Check sheet for the drawn part. Datum: minimum x, y, z corner. Units: mm. A direction names the side the tool comes from. Round coordinates to 2 decimals unless told otherwise and drop trailing zeros. Write each loop counter-clockwise with the first axis right and the second up, starting at its lowest first coordinate (ties: lowest second). Pieces come first, ordered by that corner, then holes.
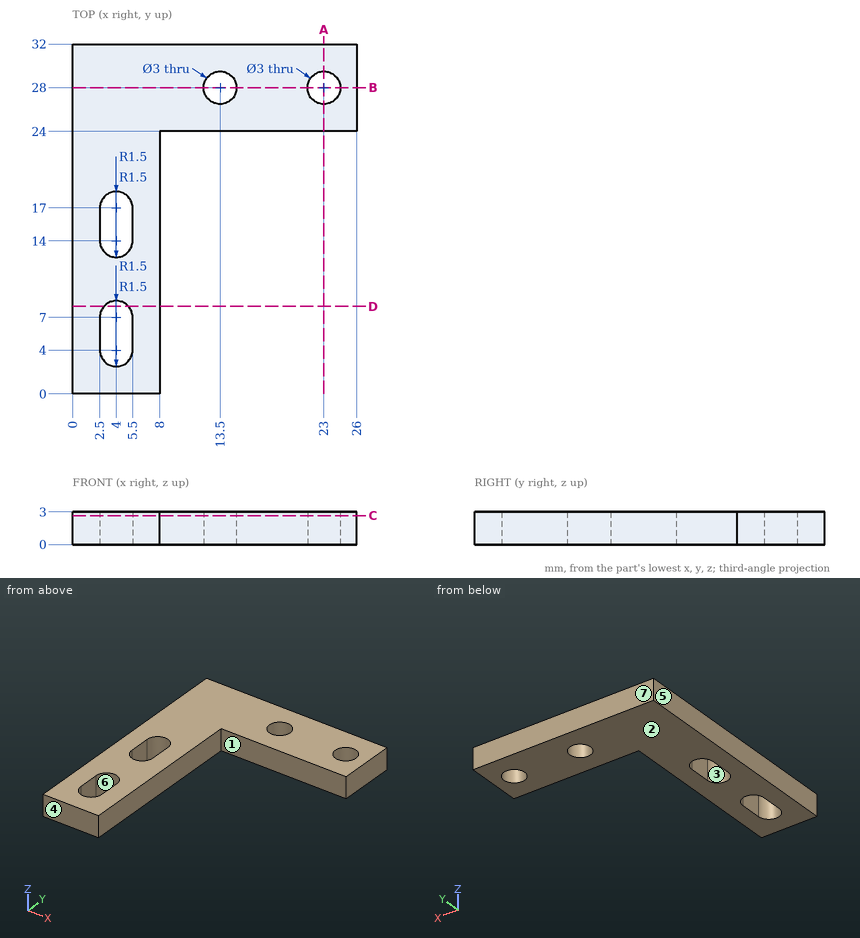
1. Release check for a two-part mould opening along Y. For the marked faces 4, 5, 6 and 7 record: released by +Y, released by -Y, zero draft, split by the parting line, or undercut.
2. Sectioned sample at A-A, the plane x = 23. Enter the section's corners in (y, z), plus the area to 3 significant figures.
3. Scan lines: line 1 along X through (y, z) = (28, 2.2); line 2 along Y through (x, z) = (13.5, 2.1); line 3 along X through (y, z) = (10, 2.25). Record each from-to range of solid material in increasing order.
4. Go/stop test with flat-tipped pins: pin 1 (3.5 mm diameter, centred on x = 13.5, y = 28, fed in from +Z); pin 2 (1.5 mm diameter, centred on y = 5.5, z = 1.5, fed in from +X). Record where each tip stops, or that it passes through.
5. Sectioned sample at B-B, the plane y = 28. Enter the section's corners in (x, z), plus the area to 3 significant figures.
6. Sectioned sample at C-C, the plane z = 2.65. Enter the section's corners in (x, y), plus the area to 3 significant figures.
7. Sectioned sample at D-D, the plane y = 8. Enter the section's corners in (x, z), plus the area to 3 significant figures.
8. Set-up check for the marked faces 1, 2 and 3: record each of +Z, -Z, +X, -X, +Y, -Y from which the full face is reachable in a straight line by a thin tool's end or side.
Computed values:
1. face 4: released by -Y
1. face 5: zero draft
1. face 6: undercut
1. face 7: released by +Y
2. outline: (24, 0) - (26.5, 0) - (26.5, 3) - (24, 3) - close; (29.5, 0) - (32, 0) - (32, 3) - (29.5, 3) - close
2. area: 15.0 mm2
3. line 1: x = 0 to 12, 15 to 21.5, 24.5 to 26
3. line 2: y = 24 to 26.5, 29.5 to 32
3. line 3: x = 0 to 8
4. pin 1: stops at z = 3
4. pin 2: stops at x = 8
5. outline: (0, 0) - (12, 0) - (12, 3) - (0, 3) - close; (15, 0) - (21.5, 0) - (21.5, 3) - (15, 3) - close; (24.5, 0) - (26, 0) - (26, 3) - (24.5, 3) - close
5. area: 60.0 mm2
6. outline: (0, 0) - (8, 0) - (8, 24) - (26, 24) - (26, 32) - (0, 32) - close; hole (2.5, 4) arc R1.5 ccw to (5.5, 4) - (5.5, 7) arc R1.5 ccw to (2.5, 7) - close; hole (2.5, 14) arc R1.5 ccw to (5.5, 14) - (5.5, 17) arc R1.5 ccw to (2.5, 17) - close; hole circle Ø3 at (13.5, 28); hole circle Ø3 at (23, 28)
6. area: 354 mm2
7. outline: (0, 0) - (2.88, 0) - (2.88, 3) - (0, 3) - close; (5.12, 0) - (8, 0) - (8, 3) - (5.12, 3) - close
7. area: 17.3 mm2
8. face 1: +Z, -Z, +X, -Y
8. face 2: -Z, +X, -X, +Y, -Y
8. face 3: +Z, -Z
